The model under review builds one solid part; all positions refer to its coordinate system, in mm. A direction names the side the tool comes from. Coordinates: 2 decimals unless noted, no trailing zeros. Write each loop counter-clockwise with the first axis right and the second up, starting at its lowest first coordinate (ties: lowest second). Pieces come first, ordered by that corner, then holes.
1) For line 1 (X direction, y = 5, z = -1.25) (3 decimals); line 2 (Z direction, x = -3, y = 6.25); line 3 (Z direction, x = -8.5, y = 0.5), list the stretches that pass through material, from the lowest coordinate up.
2) Add section C-C, the plane x = -8. State the section outline as (y, z) points, then the cut area to 3 significant figures.
3) Add section D-D, the plane z = 3.5. State the section outline as (x, y) points (3 decimals).
4) For P1, Ø2, axis at x = -11, y = -3, coming from the -Z side; P2, Ø1, axis at x = -31, z = 3.5, coming from the +Y side; P3, Ø6, axis at x = -32.5, z = 0, coming from the +Y side; P4, Ø4, axis at x = -34.5, z = -1.5, coming from the -Y side, all flat-tipped, find the tip position at first contact; note any pin that passes through.
5) Machinability: for faces 1 (the cylindrical face through (-36.75, -1.915, -1.468)), 2 (the flat face through (1.524, 0, 0)), which of the approach directions +Z, -Z, +X, -X, +Y, -Y give a long, thin tool a straight path to every point of the face, cutting with its end or side? Answer none if there is none.
6) Add section A-A, the plane y = 0. State the section outline as (x, z) points (3 decimals).
Autodesk Inventor part; units mm, degrees
ref_plane "h1_XY" through (-70.9168, 0, 0) normal (0, 1, 0) x (1, 0, 0)
ref_plane "h1_YZ" through (-70.9168, 0, 0) normal (1, 0, 0) x (0, 0, -1)
ref_plane "h1_ZX" through (-70.9168, 0, 0) normal (0, 0, -1) x (0, 1, 0)
sketch "Sketch_3" plane through (0, 0, 0) normal (0, 0, 1) x (1, 0, 0)
  line L0 (0, 0) -> (-70.9168, 0)
  line L1 (-70.9168, 0) -> (-70.9168, 1.9406)
  line L2 (-70.9168, 1.9406) -> (-70.4444, 2.413)
  line L3 (-70.4444, 2.413) -> (0, 2.413)
  line L4 (0, 2.413) -> (0, 0)
  line L5 (0, 0) -> (-70.9168, 0)
revolve "Revolution1" add sketch "Sketch_3" angle 360 about axis through (0, 0, 0) along (1, 0, 0)
thread "Thread1"
sketch "Sketch_17" plane through (0, 0, 0) normal (0, 0, 1) x (1, 0, 0)
  line L0 (70.9168, 0) -> (-70.9168, 0)
  line L1 (-58.4708, 2.413) -> (-58.4708, 2.159)
  line L2 (-58.4708, 2.159) -> (-58.2168, 2.159)
  line L3 (-58.2168, 2.159) -> (-58.2168, 2.413)
  line L4 (-58.2168, 2.413) -> (-58.4708, 2.413)
revolve "Revolution2" cut sketch "Sketch_17" angle 360 about axis through (70.9168, 0, 0) along (1, 0, 0)
sketch "Sketch_12" plane through (0, 0, 0) normal (0, 0, 1) x (1, 0, 0)
  line L0 (1.524, 0) -> (-15.875, 0)
  line L1 (-15.875, 0) -> (-15.875, 7.2771)
  line L2 (-15.875, 7.2771) -> (1.524, 7.2771)
  line L3 (1.524, 7.2771) -> (1.524, 0)
  line L4 (1.524, 0) -> (-15.875, 0)
revolve "Revolution3" add sketch "Sketch_12" angle 360 about axis through (1.524, 0, 0) along (1, 0, 0)
ref_plane "h1_XY" through (-70.9168, 0, 0) normal (0, 1, 0) x (1, 0, 0)
ref_plane "h1_YZ" through (-70.9168, 0, 0) normal (1, 0, 0) x (0, 0, -1)
ref_plane "h1_ZX" through (-70.9168, 0, 0) normal (0, 0, -1) x (0, 1, 0)
ref_plane "h2_XY" through (-58.2168, 0, 0) normal (0, 1, 0) x (1, 0, 0)
ref_plane "h2_YZ" through (-58.2168, 0, 0) normal (1, 0, 0) x (0, 0, -1)
ref_plane "h2_ZX" through (-58.2168, 0, 0) normal (0, 0, -1) x (0, 1, 0)
ref_plane "k1_XY" through (-70.9168, 0, -2.413) normal (0, 1, 0) x (1, 0, 0)
ref_plane "k1_YZ" through (-70.9168, 0, -2.413) normal (1, 0, 0) x (0, 0, -1)
ref_plane "k1_ZX" through (-70.9168, 0, -2.413) normal (0, 0, -1) x (0, 1, 0)
ref_plane "k2_XY" through (-70.9168, 0, 2.413) normal (0, 1, 0) x (1, 0, 0)
ref_plane "k2_YZ" through (-70.9168, 0, 2.413) normal (1, 0, 0) x (0, 0, -1)
ref_plane "k2_ZX" through (-70.9168, 0, 2.413) normal (0, 0, -1) x (0, 1, 0)
ref_plane "start_XY" through (-58.2168, 0, 0) normal (0, 1, 0) x (1, 0, 0)
ref_plane "start_YZ" through (-58.2168, 0, 0) normal (1, 0, 0) x (0, 0, -1)
ref_plane "start_ZX" through (-58.2168, 0, 0) normal (0, 0, -1) x (0, 1, 0)
ref_plane "to_prc_XY" through (-58.2168, 0, 0) normal (1, 0, 0) x (0, 0, -1)
ref_plane "to_prc_YZ" through (-58.2168, 0, 0) normal (0, 0, -1) x (0, 1, 0)
ref_plane "to_prc_ZX" through (-58.2168, 0, 0) normal (0, 1, 0) x (1, 0, 0)
ref_plane "to_rod_guide_XY" through (-70.9168, 0, 0) normal (1, 0, 0) x (0, 0, -1)
ref_plane "to_rod_guide_YZ" through (-70.9168, 0, 0) normal (0, 0, -1) x (0, 1, 0)
ref_plane "to_rod_guide_ZX" through (-70.9168, 0, 0) normal (0, 1, 0) x (1, 0, 0)
properties part number "D-75080.5-0.011XP-2.792-3pos"
Geometry results:
1. line 1: x = -15.875 to 1.524
1. line 2: z = -3.73 to 3.73
1. line 3: z = -7.26 to 7.26
2. outline: circle Ø14.55 at (0, 0)
2. area: 166 mm2
3. outline: (-15.875, -6.38) - (1.524, -6.38) - (1.524, 6.38) - (-15.875, 6.38) - close
4. P1: stops at z = -7
4. P2: passes through
4. P3: stops at y = 2.41
4. P4: stops at y = -2.41
5. face 1: -X
5. face 2: +Z, -Z, +X, +Y, -Y
6. outline: (-70.917, -1.941) - (-70.444, -2.413) - (-58.471, -2.413) - (-58.471, -2.159) - (-58.217, -2.159) - (-58.217, -2.413) - (-15.875, -2.413) - (-15.875, -7.277) - (1.524, -7.277) - (1.524, 7.277) - (-15.875, 7.277) - (-15.875, 2.413) - (-58.217, 2.413) - (-58.217, 2.159) - (-58.471, 2.159) - (-58.471, 2.413) - (-70.444, 2.413) - (-70.917, 1.941) - close
